Input: part model. Units: mm. Frame: model coordinates. A direction names the side the tool comes from. Round coordinates to 2 decimals unless told otherwise and drop trailing zeros. Loops run counter-clockwise (first coordinate to the right, second up) from the corner with the lowest first, then second, coordinate; pieces in that order, holes last. Notation, with made-up numbers: (24.5, -2.5) -> (76.5, -2.5) arc R22 cw to (76.5, 24.5) -> close; hole circle Ø2 at (-14, 41.25). An arc over 180 degrees is marked (long way). Answer as a JSON object with one key per item and string values.
```python
from build123d import *

# Parameters (mm, degrees)
SKETCH1_R           = 75
BOSS_EXTRUDE3_DEPTH = 19.2
SKETCH3_R           = 70
CUT_EXTRUDE1_DEPTH  = 9.6
SKETCH4_R           = 30
BOSS_EXTRUDE4_DEPTH = 30
SKETCH5_R           = 15
CUT_EXTRUDE2_DEPTH  = 57
SKETCH6_R           = 4
CUT_EXTRUDE3_DEPTH  = 57
SKETCH7_W           = 8
SKETCH7_H           = 10
CUT_EXTRUDE4_DEPTH  = 30


with BuildPart() as part:
    # Sketch1 → Boss-Extrude3 (new body)
    with BuildSketch(Plane.XY):
        Circle(SKETCH1_R)
    extrude(amount=BOSS_EXTRUDE3_DEPTH)

    # Sketch3 → Cut-Extrude1 (cut)
    with BuildSketch(Plane.XY.offset(19.2)):
        Circle(SKETCH3_R)
    extrude(amount=-CUT_EXTRUDE1_DEPTH, mode=Mode.SUBTRACT)

    # Sketch4 → Boss-Extrude4 (add)
    with BuildSketch(Plane.XY.offset(9.6)):
        Circle(SKETCH4_R)
    extrude(amount=BOSS_EXTRUDE4_DEPTH)

    # Sketch5 → Cut-Extrude2 (cut)
    with BuildSketch(Plane.XY.offset(39.6)):
        Circle(SKETCH5_R)
    extrude(amount=-CUT_EXTRUDE2_DEPTH, mode=Mode.SUBTRACT)

    # Sketch6 → Cut-Extrude3 (cut)
    with BuildSketch(Plane.XY.offset(9.6)):
        with Locations((0, 60)):
            Circle(SKETCH6_R)
        with Locations((60, 0)):
            Circle(SKETCH6_R)
        with Locations((0, -60)):
            Circle(SKETCH6_R)
        with Locations((-60, 0)):
            Circle(SKETCH6_R)
    extrude(amount=-CUT_EXTRUDE3_DEPTH, mode=Mode.SUBTRACT)

    # Sketch7 → Cut-Extrude4 (cut)
    with BuildSketch(Plane.XY.offset(39.6)):
        with Locations((0, 15)):
            Rectangle(SKETCH7_W, SKETCH7_H)
    extrude(amount=-CUT_EXTRUDE4_DEPTH, mode=Mode.SUBTRACT)


solid = part.part
```
1) Section B-B, the plane y = 0. Output: boundary loops of the cut face in (x, z).
Output:
{"outline": "(-75, 0) -> (-64, 0) -> (-64, 9.6) -> (-70, 9.6) -> (-70, 19.2) -> (-75, 19.2) -> close; (-56, 0) -> (-15, 0) -> (-15, 39.6) -> (-30, 39.6) -> (-30, 9.6) -> (-56, 9.6) -> close; (15, 0) -> (56, 0) -> (56, 9.6) -> (30, 9.6) -> (30, 39.6) -> (15, 39.6) -> close; (64, 0) -> (75, 0) -> (75, 19.2) -> (70, 19.2) -> (70, 9.6) -> (64, 9.6) -> close"}
2) Ray query, probe 1 along Y at (x, z) = (0, 2.5); probe 2 along X at (y, z) = (-18.5, 16.5); probe 3 along Z at (x, y) = (-11, -43.5). Return the intervals inside material, ascending.
Output:
{"probe 1": "y = -75 to -64, -56 to -15, 15 to 56, 64 to 75", "probe 2": "x = -72.68 to -67.51, -23.62 to 23.62, 67.51 to 72.68", "probe 3": "z = 0 to 9.6"}
3) Contact query for flat-ended pins moving along their axis: P1, Ø2.5, axis at x = -1, z = 26.5, coming from the -Y side; P2, Ø4, axis at y = -42.5, z = 13, coming from the -X side; P3, Ø8, axis at y = 23.5, z = 27, coming from the +X side; P4, Ø5, axis at y = -47.5, z = 23, coming from the +X side. Output: stop coordinate, or through.
Output:
{"P1": "stops at y = -30", "P2": "stops at x = -63.12", "P3": "stops at x = 22.8", "P4": "passes through"}
4) Section D-D, the plane x = -60. Output: boundary loops of the cut face in (y, z), plus the area to 3 significant figures.
Output:
{"outline": "(-45, 0) -> (-4, 0) -> (-4, 9.6) -> (-36.06, 9.6) -> (-36.06, 19.2) -> (-45, 19.2) -> close; (4, 0) -> (45, 0) -> (45, 19.2) -> (36.06, 19.2) -> (36.06, 9.6) -> (4, 9.6) -> close", "area": "959 mm^2"}
5) Draft query along X for faces 1 (the face through (-3.252, -14.643, 20.077)), 2 (the face through (-9.764, 74.362, 9.466)), 3 (the face through (6, 14, 39.6)), 4 (the face through (0, 17, 9.6)). Return one class per face: +X half, -X half, draft (parallel to the pull), parting line (faces both ways), or undercut.
Output:
{"face 1": "undercut", "face 2": "parting line", "face 3": "draft", "face 4": "undercut"}
6) Reachability of faces 5 (the face through (-55.55, -42.594, 14.467)), 6 (the face through (-0.867, 56.095, 4.867)) from +Z, -Z, +X, -X, +Y, -Y: full face, straight path, thin tool, end or side. Return the list, or none.
Output:
{"face 5": "+Z", "face 6": "+Z, -Z"}
7) Section C-C, the plane z = 4. Output: boundary loops of the cut face in (x, y).
Output:
{"outline": "circle Ø150 at (0, 0); hole circle Ø8 at (-60, 0); hole circle Ø30 at (0, 0); hole circle Ø8 at (0, -60); hole circle Ø8 at (0, 60); hole circle Ø8 at (60, 0)"}
8) Section A-A, the plane z = 16.5. Output: boundary loops of the cut face in (x, y), plus the area to 3 significant figures.
Output:
{"outline": "circle Ø150 at (0, 0); circle Ø60 at (0, 0); hole circle Ø140 at (0, 0); hole (-4, 14.46) arc R15 ccw (long way) to (4, 14.46) -> (4, 20) -> (-4, 20) -> close", "area": "4,360 mm^2"}
